Could you check a few things on this model? Use its own coordinates, in mm. Coordinates: 2 decimals unless noted, no trailing zeros. Order: outer loops, then holes, each group sorted by start corner. A loop starts at its lowest first (then second) coordinate and runs counter-clockwise, first axis right, second up. Notation, with made-up numbers: M 3.25,40.5 L 23.25,40.5 A22 cw 23.25,76.5 Z; hole C -8,-9 d9. An arc over 180 degrees is marked long. Put each result on its own line as item: value. Start each with the question number.
```python
from build123d import *

# Parameters (mm, degrees)
F0_W     = 50.8
F0_H     = 50.8
F0_R     = 11.259626
F1_DEPTH = 25.4


with BuildPart() as f1:
    # F0 (on Top) → F1 (new body)
    with BuildSketch(Plane.XY):
        with Locations((3.039317, 5.644446)):
            Rectangle(F0_W, F0_H)
        Circle(F0_R, mode=Mode.SUBTRACT)
    extrude(amount=-F1_DEPTH)


solid = f1.part
```
Item 1: If we section it at A-A on y = 0: Write out the boundary of the cut face in (x, z), then the cut area to 3 significant figures.
Item 2: If we section it at B-B on x = -6: Write out the boundary of the cut face in (y, z).
Item 3: If we mould it in two halves opening along X, with no side actions, what happens to faces 1 (the cylindrical face through (-8.9, -6.9, -12.5)), 2 (the flat face through (3, 12, -25.4)), 3 (the flat face through (-22.361, 5, -13))? For each: released by +X, released by -X, zero draft, split by the parting line, or undercut.
Item 4: I need wall thicknesses on probe 1 along Y at (x, z) = (0, -12.75); probe 2 along X at (y, z) = (6.5, -7.5); probe 3 along Y at (x, z) = (-10, -9.5). Which ranges of each line are inside material? Lowest first, please.
Item 5: If we section it at C-C on z = -2.25: Write out the boundary of the cut face in (x, y), then the cut area to 3 significant figures.
Geometry check:
1. outline: M -22.36,-25.4 L -11.26,-25.4 L -11.26,0 L -22.36,0 Z; M 11.26,-25.4 L 28.44,-25.4 L 28.44,0 L 11.26,0 Z
1. area: 718 mm²
2. outline: M -19.76,-25.4 L -9.53,-25.4 L -9.53,0 L -19.76,0 Z; M 9.53,-25.4 L 31.04,-25.4 L 31.04,0 L 9.53,0 Z
3. face 1: undercut
3. face 2: zero draft
3. face 3: released by -X
4. probe 1: y = -19.76 to -11.26, 11.26 to 31.04
4. probe 2: x = -22.36 to -9.19, 9.19 to 28.44
4. probe 3: y = -19.76 to -5.17, 5.17 to 31.04
5. outline: M -22.36,-19.76 L 28.44,-19.76 L 28.44,31.04 L -22.36,31.04 Z; hole C 0,0 d22.52
5. area: 2,180 mm²
